The listing builds one solid part. Answer for the finished solid, in the listing's coordinates (mm). Face numbers are marked on the shaded views. A direction names the side the tool comes from. Coordinates: 2 decimals unless noted, no trailing zeros. Order: outer loops, then holes, each group sorted by start corner. A loop starts at its lowest first (then second) coordinate and runs counter-clockwise, first axis right, second up. Notation, with made-up numbers: M 88,-20.75 L 121,-20.75 A17 cw 121,11.25 Z; hole C -38,-15.5 d9. An arc over 180 degrees is marked long. One line per item, written item: value. Start each with the question number.
Q1. Straight lines are drawn through the part: line 1 along X through (y, z) = (100.5, -107); line 2 along Y through (x, z) = (12, -55.5). For each, find the intervals that lie inside material, in ascending order. Write a range as [from, to].
Q2. Each of these flat-tipped pins is pushed along its axis until it touches: pin 1 Ø1 at (y, z) = (92, -15) entering from -X; pin 2 Ø8 at (x, y) = (43.5, 54.5) entering from +Z; pin 3 Ø23 at (x, z) = (16.5, -31) entering from +Y. Where does it stop, or does it pass through?
Q3. The part is cut by section B-B on x = 41. Give the vertices of the cut face in (y, z), then the cut area to 3 significant figures.
Q4. The part is cut by section C-C on y = 36. Give the vertices of the cut face in (x, z), then the cut area to 3 significant figures.
Q5. The part is cut by section A-A on z = -51. Give the vertices of the cut face in (x, y), then the cut area to 3 significant figures.
Q6. For the marked faces 1 and 2, determine the directions among +Z, -Z, +X, -X, +Y, -Y from which every point of the face is accessible in a straight line to the end or side of a thin tool.
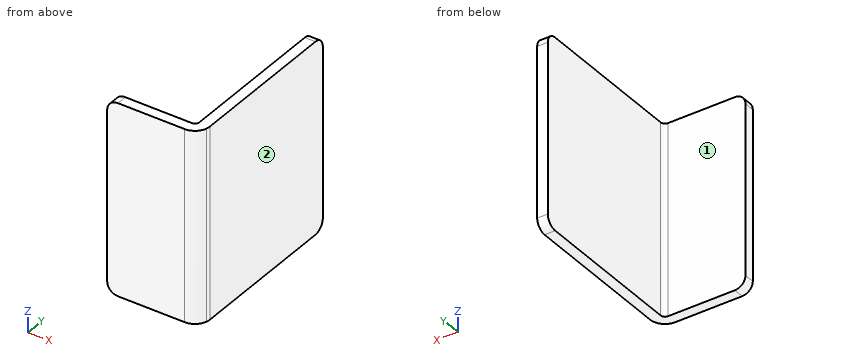
```python
from build123d import *

# Parameters (mm, degrees)
SKETCH11_W             = 152.4
SKETCH11_H             = 114.3
BOSS_EXTRUDE1_DEPTH    = 6.35
SKETCHED_START         = -114.3
SKETCHED_BEND1_DEPTH   = 114.3
SKETCHED_BEND1_2_DEPTH = 114.3
FILLET1_R              = 6.35


# Read off the part's stored shape, not the designer's step: Sketched Bend1
with BuildPart() as part:
    # Sketch11 → Boss-Extrude1 (new body)
    with BuildSketch(Plane(origin=(0, 0, 0), x_dir=(1, 0, 0), z_dir=(0, 1, 0))):
        with Locations((76.2, 57.15)):
            Rectangle(SKETCH11_W, SKETCH11_H)
    extrude(amount=BOSS_EXTRUDE1_DEPTH)

    # Sketched Bend1 outline → Sketched Bend1 (cut)
    with BuildSketch(Plane.XY.offset(SKETCHED_START)):
        with BuildLine():
            Line((152.4, 6.35), (54.83086849, 6.35))
            ThreePointArc((54.83086849, 6.35), (51.624240665, 1.762142678), (46.311449496, 0))
            Line((46.311449496, 0), (152.4, 0))
            Line((152.4, 0), (152.4, 6.35))
        make_face()
    extrude(amount=SKETCHED_BEND1_DEPTH, mode=Mode.SUBTRACT)

    # Sketched Bend1 2 outline → Sketched Bend1 2 (add)
    with BuildSketch(Plane.XY.offset(SKETCHED_START)):
        with BuildLine():
            Line((48.851449496, 106.001449496), (48.851449496, 8.89))
            ThreePointArc((48.851449496, 8.89), (48.10750072, 7.093948776), (46.311449496, 6.35))
            Line((46.311449496, 6.35), (54.83086849, 6.35))
            ThreePointArc((54.83086849, 6.35), (55.108316406, 7.606554415), (55.201449496, 8.89))
            Line((55.201449496, 8.89), (55.201449496, 106.001449496))
            Line((55.201449496, 106.001449496), (48.851449496, 106.001449496))
        make_face()
    extrude(amount=SKETCHED_BEND1_2_DEPTH)

    # Fillet1
    fillet1_edges = [part.edges().sort_by_distance(p)[0] for p in [
        (0, 3.175, 0),
        (0, 3.175, -114.3),
        (52.026449496, 106.001449496, -114.3),
        (52.026449496, 106.001449496, 0),
    ]]
    fillet(fillet1_edges, radius=FILLET1_R)


solid = part.part
```
Output:
1. line 1: x = [48.85, 55.2]
1. line 2: y = [0, 6.35]
2. pin 1: stops at x = 48.85
2. pin 2: passes through
2. pin 3: stops at y = 6.35
3. outline: M 0,-114.3 L 6.35,-114.3 L 6.35,0 L 0,0 Z
3. area: 726 mm^2
4. outline: M 48.85,-114.3 L 55.2,-114.3 L 55.2,0 L 48.85,0 Z
4. area: 726 mm^2
5. outline: M 0,0 L 46.31,0 A8.89 ccw 55.2,8.89 L 55.2,106 L 48.85,106 L 48.85,8.89 A2.54 cw 46.31,6.35 L 0,6.35 Z
5. area: 968 mm^2
6. face 1: +Z, -Z, -X, +Y
6. face 2: +Z, -Z, +X, +Y, -Y
